The figure shows three views and two pictorial views of one solid part (mm, origin at its lowest corner). Answer the questions. A direction names the side the tool comes from. Coordinates: 2 decimals unless noted, no trailing zeros. Loops run counter-clockwise (first coordinate to the right, second up) from the corner with the lowest first, then second, coordinate; pieces in that order, holes last. Notation, with made-up numbers: M 40,-9 L 73,-9 A22 cw 73,2 Z; hole C 38.25,22.25 d6. An arc over 180 degrees is marked long. Answer as a JSON object with one key per item and string values. Group by question number.
1. Given pin 1 (3.5 mm diameter, centred on x = 6, y = 35.5, fed in from +Z); pin 2 (12 mm diameter, centred on x = 48.5, y = 38, fed in from +Z); pin 3 (0.8 mm diameter, centred on y = 30.5, z = 4.5, fed in from -X); pin 4 (6 mm diameter, centred on x = 5.5, y = 16, fed in from -Z), each flat-ended and moving along its own axis, determine where each tip first touches the part or whether it passes through.
2. A cutting plane is placed at A-A on x = 5.5. Give the vertices of the cut face in (y, z).
3. For the marked faces 1, 2 and 3, determine the directions among +Z, -Z, +X, -X, +Y, -Y from which every point of the face is accessible in a straight line to the end or side of a thin tool.
4. Straight lines are drawn through the part: L1, parallel to Y at x = 5.5, z = 1; L2, parallel to Y at x = 51, z = 2.8; L3, parallel to Z at x = 45.5, y = 47. For each, find the intervals that lie inside material, in ascending order.
5. A cutting plane is placed at B-B on y = 38. Give the vertices of the cut face in (x, z), and give its area (3 significant figures).
6. A cutting plane is placed at C-C on z = 3.3. Give the vertices of the cut face in (x, y), and give its area (3 significant figures).
7. A cutting plane is placed at D-D on y = 15. Give the vertices of the cut face in (x, z), and give its area (3 significant figures).
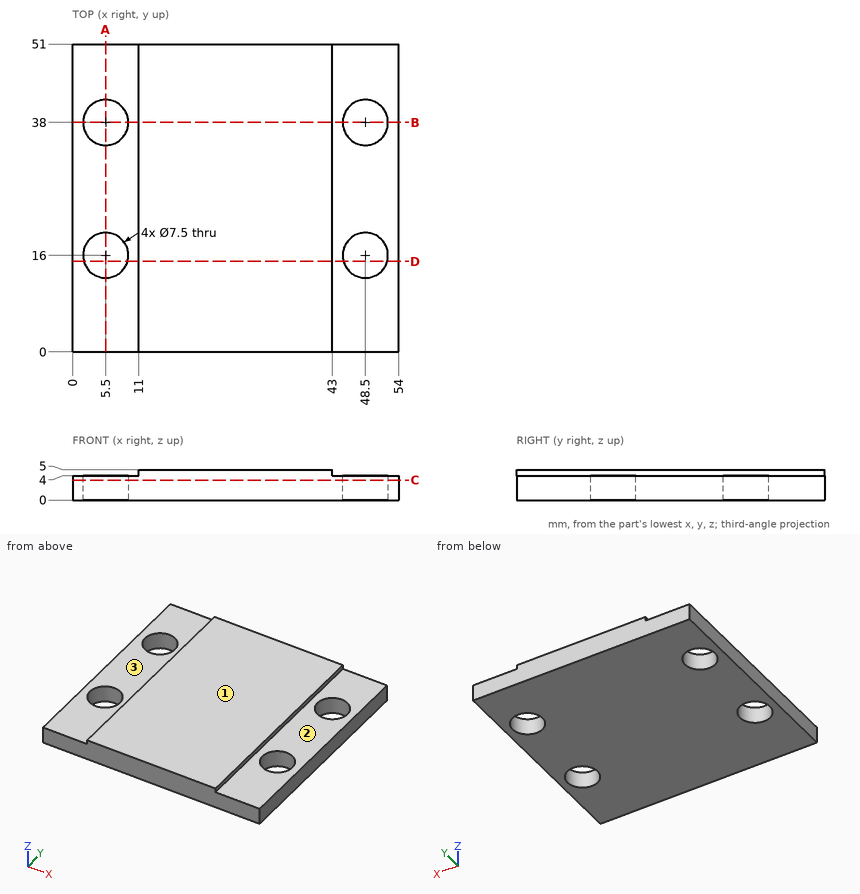
From the geometry:
{
 "1": {"pin 1": "stops at z = 4", "pin 2": "stops at z = 5", "pin 3": "stops at x = 11", "pin 4": "passes through"},
 "2": {"outline": "M 0,0 L 12.25,0 L 12.25,4 L 0,4 Z; M 19.75,0 L 34.25,0 L 34.25,4 L 19.75,4 Z; M 41.75,0 L 51,0 L 51,4 L 41.75,4 Z"},
 "3": {"face 1": "+Z, +X, -X, +Y, -Y", "face 2": "+Z, +X, +Y, -Y", "face 3": "+Z, -X, +Y, -Y"},
 "4": {"L1": "y = 0 to 12.25, 19.75 to 34.25, 41.75 to 51", "L2": "y = 0 to 13.2, 18.8 to 35.2, 40.8 to 51", "L3": "z = 0 to 4"},
 "5": {"outline": "M 0,0 L 1.75,0 L 1.75,4 L 0,4 Z; M 9.25,0 L 44.75,0 L 44.75,4 L 43,4 L 43,5 L 11,5 L 11,4 L 9.25,4 Z; M 52.25,0 L 54,0 L 54,4 L 52.25,4 Z", "area": "188 mm²"},
 "6": {"outline": "M 0,0 L 54,0 L 54,51 L 0,51 Z; hole C 5.5,16 d7.5; hole C 5.5,38 d7.5; hole C 48.5,16 d7.5; hole C 48.5,38 d7.5", "area": "2,580 mm²"},
 "7": {"outline": "M 0,0 L 1.89,0 L 1.89,4 L 0,4 Z; M 9.11,0 L 44.89,0 L 44.89,4 L 43,4 L 43,5 L 11,5 L 11,4 L 9.11,4 Z; M 52.11,0 L 54,0 L 54,4 L 52.11,4 Z", "area": "190 mm²"}
}
